from build123d import *

# Parameters (mm, degrees)
SCHIZZO2_R                   = 5
SCHIZZO2_R_2                 = 3
ESTRUSIONE_ESTRUSIONE1_DEPTH = 1.25
RACCORDO4_R                  = 0.9


with BuildPart() as part:
    # Schizzo1 → Rivoluzione8 (revolve)
    with BuildSketch(Plane.XY):
        with BuildLine():
            Line((0, -15), (0, 15))
            ThreePointArc((0, 15), (-15, 0), (0, -15))
        make_face()
    revolve(axis=Axis((0, 32.442859412, 0), (0, -1, 0)))

    # Schizzo2 → Estrusione-Estrusione1 (add, symmetric)
    with BuildSketch(Plane.XY):
        with Locations((0, 19.00431954)):
            Circle(SCHIZZO2_R)
        with Locations((0, 19.00431954)):
            Circle(SCHIZZO2_R_2, mode=Mode.SUBTRACT)
    extrude(amount=ESTRUSIONE_ESTRUSIONE1_DEPTH, both=True)

    # Raccordo4
    raccordo4_edges = [part.edges().sort_by_distance(p)[0] for p in [
        (-3, 19.00431954, 1.25),
        (-3, 19.00431954, -1.25),
        (0, 24.00431954, -1.25),
        (0, 24.00431954, 1.25),
    ]]
    fillet(raccordo4_edges, radius=RACCORDO4_R)


solid = part.part
Input: part model. Units: mm. Frame: model coordinates. Coordinates: 2 decimals unless noted, no trailing zeros. Order: outer loops, then holes, each group sorted by start corner. A loop starts at its lowest first (then second) coordinate and runs counter-clockwise, first axis right, second up. Notation, with made-up numbers: M 58.5,-21 L 78.5,-21 A20 ccw 78.5,-2 Z; hole C 10.25,20 d4. An arc over 180 degrees is marked long. Answer as CSV lines item,"result".
1. Section A-A (x = 0). Return the cut outline in (y, z), then the cut area to 3 significant figures.
Reported:
outline,"M 14.95,-1.25 L 15.1,-1.25 A0.9 ccw 16,-0.35 L 16,0.35 A0.9 ccw 15.1,1.25 L 14.95,1.25 A15 ccw long Z; M 22,-0.35 A0.9 ccw 22.9,-1.25 L 23.1,-1.25 A0.9 ccw 24,-0.35 L 24,0.35 A0.9 ccw 23.1,1.25 L 22.9,1.25 A0.9 ccw 22,0.35 Z"
area,"713 mm2"
2. First-contact query: P1, Ø6, axis at x = 2.5, z = -8, coming from the +Y side; P2, Ø12, axis at x = 6.5, y = 3, coming from the -Z side; P3, Ø12, axis at x = -9.5, z = 2.5, coming from the +Y side; P4, Ø3.5, axis at x = 0, y = 19, coming from the -Z side. Flat tips, straight axial feed; report the tip coordinate or a pass-through.
Reported:
P1,"y = 14"
P2,"z = -14.96"
P3,"y = 22.19"
P4,"through"
3. Section B-B (y = -11.5). Return the cut outline in (x, z), then the cut area to 3 significant figures.
Reported:
outline,"C 0,0 d19.26"
area,"291 mm2"
4. Section C-C (z = -3.5). Return the cut outline in (x, y).
Reported:
outline,"C 0,0 d29.17"
5. Material intervals for line 1 (Y direction, x = 0, z = 0.2); line 2 (X direction, y = 20.5, z = 0.75); line 3 (Y direction, x = 1.25, z = -6), sorted ascending. Write a range as from..to.
Reported:
line 1,"-15..16, 22..24"
line 2,"-4.67..-2.71, 2.71..4.67"
line 3,"-13.69..13.69"
